Build history of the part. All positions in model axes, mm. Face numbers are marked on the shaded views. Coordinates: 2 decimals unless noted, no trailing zeros. Write each loop counter-clockwise with the first axis right and the second up, starting at its lowest first coordinate (ties: lowest second). Pieces come first, ordered by that corner, then holes.
```python
from build123d import *

# Parameters (mm, degrees)
SKETCH1_W           = 76.2
SKETCH1_H           = 50.8
SKETCH1_R           = 4.31365531
BOSS_EXTRUDE2_DEPTH = 25.4
SKETCH6_R           = 4.1275
SKETCH6_R_2         = 3.175
CUT_EXTRUDE3_DEPTH  = 25.4


with BuildPart() as part:
    # Sketch1 → Boss-Extrude2 (new body)
    with BuildSketch(Plane.XY):
        with Locations((38.1, 25.4)):
            Rectangle(SKETCH1_W, SKETCH1_H)
        with Locations((38.1, 38.1)):
            Circle(SKETCH1_R, mode=Mode.SUBTRACT)
        with Locations((50.8, 25.4)):
            Circle(SKETCH1_R, mode=Mode.SUBTRACT)
        with Locations((38.1, 12.7)):
            Circle(SKETCH1_R, mode=Mode.SUBTRACT)
        with Locations((25.4, 25.4)):
            Circle(SKETCH1_R, mode=Mode.SUBTRACT)
    extrude(amount=BOSS_EXTRUDE2_DEPTH)

    # Sketch6 → Cut-Extrude3 (cut)
    with BuildSketch(Plane.XY.offset(25.4)):
        with Locations((38.1, 25.4)):
            Circle(SKETCH6_R)
        with Locations((6.35, 44.45)):
            Circle(SKETCH6_R_2)
        with Locations((69.85, 44.45)):
            Circle(SKETCH6_R_2)
        with Locations((6.35, 6.35)):
            Circle(SKETCH6_R_2)
        with Locations((69.85, 6.35)):
            Circle(SKETCH6_R_2)
    extrude(amount=-CUT_EXTRUDE3_DEPTH, mode=Mode.SUBTRACT)


solid = part.part
```
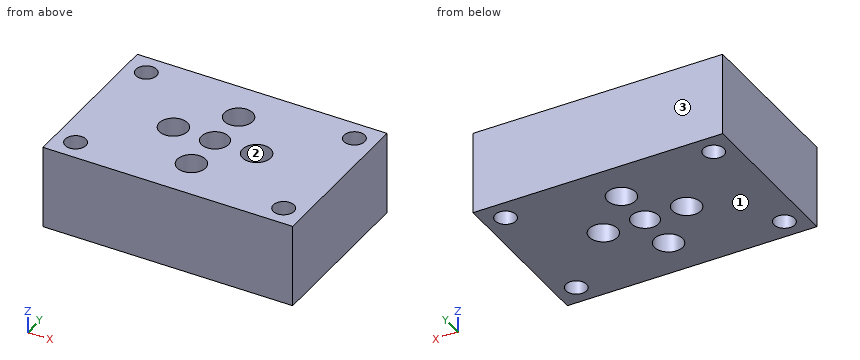
1. Saw through at B-B on x = 50.8. List the corners of the cut face in (y, z), plus the area to 3 significant figures.
Computed values:
outline: (0, 0) - (21.09, 0) - (21.09, 25.4) - (0, 25.4) - close; (29.71, 0) - (50.8, 0) - (50.8, 25.4) - (29.71, 25.4) - close
area: 1,070 mm2
2. Saw through at C-C on z = 3. State how many separate pieces and enclosed holes the cut face has, plus the area to 3 significant figures.
Computed values:
separate pieces: 1
enclosed holes: 9
area: 3,460 mm2
3. Flat gauge pin, fed straight in: pin 1 (8 mm diameter, centred on x = 50.8, y = 25.4, fed in from +Z). Where does the tip first touch, or does it go through?
Computed values:
pin 1: passes through
4. Saw through at A-A on y = 25.4. List the corners of the cut face in (x, z), plus the area to 3 significant figures.
Computed values:
outline: (0, 0) - (21.09, 0) - (21.09, 25.4) - (0, 25.4) - close; (29.71, 0) - (33.97, 0) - (33.97, 25.4) - (29.71, 25.4) - close; (42.23, 0) - (46.49, 0) - (46.49, 25.4) - (42.23, 25.4) - close; (55.11, 0) - (76.2, 0) - (76.2, 25.4) - (55.11, 25.4) - close
area: 1,290 mm2
5. Probe line 1 along Y through (x, z) = (38.1, 18.5); line 2 along X through (y, z) = (6, 18.5); line 3 along X through (y, z) = (27.5, 1.25). List the from-to ranges inside material, lowest first.
Computed values:
line 1: y = 0 to 8.39, 17.01 to 21.27, 29.53 to 33.79, 42.41 to 50.8
line 2: x = 0 to 3.19, 9.51 to 66.69, 73.01 to 76.2
line 3: x = 0 to 21.63, 29.17 to 34.55, 41.65 to 47.03, 54.57 to 76.2
6. Saw through at D-D on x = 69.85. List the corners of the cut face in (y, z) (3 decimals), plus the area to 3 significant figures.
Computed values:
outline: (0, 0) - (3.175, 0) - (3.175, 25.4) - (0, 25.4) - close; (9.525, 0) - (41.275, 0) - (41.275, 25.4) - (9.525, 25.4) - close; (47.625, 0) - (50.8, 0) - (50.8, 25.4) - (47.625, 25.4) - close
area: 968 mm2
7. Mould opens along Y. For the marked faces 1, 2 and 3 say: +Y half, -Y half, draft (parallel to the pull), parting line (faces both ways), or undercut.
Computed values:
face 1: draft
face 2: undercut
face 3: +Y half
